Check sheet for the modelled part. Datum: model origin and axes. Units: mm. A direction names the side the tool comes from. Give positions to 0.01 mm unless a question says otherwise; leave off trailing zeros. Write each loop counter-clockwise with the first axis right and the second up, starting at its lowest first coordinate (ties: lowest second). Pieces come first, ordered by that corner, then holes. Notation, with made-up numbers: M 3.5,86 L 20.5,86 A21 cw 20.5,122 Z; hole C 70.25,-24 d4. An arc over 180 degrees is marked long. Write item = value, one per line. Start each with the question number.
1) Cross-section at A-A, the plane x = 36.5. Record the cut outline in (y, z), plus the area to 4 significant figures.
2) Access from +Z, -Z, +X, -X, +Y, -Y to the whole of each face (thin tool, end or side, straight path). Record for faces 1 (the flat face through (28, 39.5, -2)), 2 (the flat face through (27, 5.5, -2)), 3 (the flat face through (44.5, 22, -2)).
3) Cross-section at D-D, the plane y = 22.5. Record the cut outline in (x, z).
4) Cross-section at B-B, the plane y = 10. Record the cut outline in (x, z), plus the area to 3 significant figures.
5) Go/stop test with flat-tipped pins: pin 1 (1.5 mm diameter, centred on y = 23, z = -3, fed in from -X); pin 2 (2 mm diameter, centred on y = 33, z = -0.5, fed in from +X); pin 3 (1 mm diameter, centred on x = 46, y = 15, fed in from -Z); pin 4 (2.5 mm diameter, centred on y = 16.5, z = -2, fed in from +X). Record where each tip stops, or that it passes through.
6) Cross-section at C-C, the plane z = -2.75. Record the cut outline in (x, y).
7) Scan lines: line 1 along X through (y, z) = (10, -1.75); line 2 along X through (y, z) = (10, 2); line 3 along Y through (x, z) = (18.5, 0.5). Record each from-to range of solid material in increasing order. Write a range as [from, to].
Solid Edge part; units mm, degrees
sketch "Sketch1" plane through (0, 0, 0) normal (0, 0, 1) x (1, 0, 0)
  line L0 (55, 0) -> (55, 45)
  line L1 (55, 45) -> (0, 45)
  line L2 (0, 45) -> (0, 0)
  line L3 (0, 0) -> (55, 0)
extrude "Protrusion1" add sketch "Sketch1" along normal blind 4
sketch "Sketch2" plane through (22.5, 22.5, 0) normal (0, 0, -1) x (1, 0, 0)
  line L0 (-12, 17) -> (22, 17)
  line L1 (22, 17) -> (22, -17)
  line L2 (22, -17) -> (-12, -17)
  line L3 (-12, -17) -> (-12, 17)
extrude "ExtrudedProtrusion_2" add sketch "Sketch2" along normal blind 5
hole "Hole_1" at (18.5, 10, 4) direction (0, 0, -1) diameter 2.5 depth 10
hole "Hole1" at (36.5, 10, 4) direction (0, 0, -1) diameter 2.5 depth 10
Reply:
q1.outline = M 0,0 L 5.5,0 L 5.5,-5 L 8.75,-5 L 8.75,4 L 0,4 Z; M 11.25,-5 L 39.5,-5 L 39.5,0 L 45,0 L 45,4 L 11.25,4 Z
q1.area = 327.5 mm2
q2.face_1 = -Z, +X, -X, +Y
q2.face_2 = -Z, +X, -X, -Y
q2.face_3 = -Z, +X, +Y, -Y
q3.outline = M 0,0 L 10.5,0 L 10.5,-5 L 44.5,-5 L 44.5,0 L 55,0 L 55,4 L 0,4 Z
q4.outline = M 0,0 L 10.5,0 L 10.5,-5 L 17.25,-5 L 17.25,4 L 0,4 Z; M 19.75,-5 L 35.25,-5 L 35.25,4 L 19.75,4 Z; M 37.75,-5 L 44.5,-5 L 44.5,0 L 55,0 L 55,4 L 37.75,4 Z
q4.area = 345 mm2
q5.pin_1 = 10.5
q5.pin_2 = 55
q5.pin_3 = 0
q5.pin_4 = 44.5
q6.outline = M 10.5,5.5 L 44.5,5.5 L 44.5,39.5 L 10.5,39.5 Z; hole C 18.5,10 d2.5; hole C 36.5,10 d2.5
q7.line_1 = [10.5, 17.25], [19.75, 35.25], [37.75, 44.5]
q7.line_2 = [0, 17.25], [19.75, 35.25], [37.75, 55]
q7.line_3 = [0, 8.75], [11.25, 45]
